```python
from build123d import *

# Parameters (mm, degrees)
ESQUISSE1_W                   = 32
ESQUISSE1_H                   = 100
BOSS_EXTRU_1_DEPTH            = 4
CHANFREIN1_SIZE               = 2.5
ESQUISSE2_W                   = 18
ESQUISSE2_H                   = 45
BOSS_EXTRU_2_DEPTH            = 32
ENL_V_MAT_EXTRU_1_DEPTH       = 151.159914758
ENL_V_MAT_EXTRU_1_DEPTH_BACK  = 151.159914758
ESQUISSE3_R                   = 3.25
ENL_V_MAT_EXTRU_2_DEPTH       = 143.91256068
ENL_V_MAT_EXTRU_2_DEPTH_BACK  = 143.91256068
ESQUISSE4_W                   = 55
ESQUISSE4_H                   = 32
ENL_V_MAT_EXTRU_3_DEPTH       = 117.292734081
ENL_V_MAT_EXTRU_3_DEPTH_BACK  = 117.292734081
ESQUISSE5_W                   = 45
ESQUISSE5_H                   = 23.5
CHANFREIN2_SIZE               = 6.5
ENL_V_MAT_EXTRU_4_DEPTH       = 5
ENL_V_START                   = 50
ENL_V_MAT_EXTRU_6_DEPTH       = 5
CONG_2_R                      = 3
ENL_V_MAT_EXTRU_7_DEPTH       = 151.159914758
ENL_V_MAT_EXTRU_7_DEPTH_BACK  = 151.159914758
CONG_3_R                      = 8
BOSS_EXTRU_3_DEPTH            = 4
BOSS_EXTRU_4_DEPTH            = 68
ESQUISSE10_W                  = 45
ESQUISSE10_H                  = 10
ENL_V_MAT_EXTRU_8_DEPTH       = 143.070405081
ENL_V_MAT_EXTRU_9_DEPTH       = 143.070405081
ENL_V_MAT_EXTRU_9_DEPTH_BACK  = 143.070405081
ESQUISSE11_R                  = 2.75
ENL_V_MAT_EXTRU_10_DEPTH      = 143.91256068
ENL_V_MAT_EXTRU_10_DEPTH_BACK = 143.91256068
ESQUISSE12_W                  = 24
ESQUISSE12_H                  = 5
CONG_4_R                      = 10
CONG_5_R                      = 3


# Some blends are built 0.0001 mm under size
with BuildPart() as part:
    # Esquisse1 → Boss.-Extru.1 (new body)
    with BuildSketch(Plane.XY):
        with Locations((16, 50)):
            Rectangle(ESQUISSE1_W, ESQUISSE1_H)
    extrude(amount=BOSS_EXTRU_1_DEPTH)

    # Chanfrein1
    chanfrein1_edges = [part.edges().sort_by_distance(p)[0] for p in [
        (16, 0, 0),
    ]]
    chamfer(chanfrein1_edges, length=CHANFREIN1_SIZE)

    # Esquisse2 → Boss.-Extru.2 (add)
    with BuildSketch(Plane(origin=(0, 0, 0), x_dir=(-1, 0, 0), z_dir=(0, 0, -1))):
        with Locations((-41, 107.5)):
            Rectangle(ESQUISSE2_W, ESQUISSE2_H)
        with Locations((9, 107.5)):
            Rectangle(ESQUISSE2_W, ESQUISSE2_H)
    extrude(amount=-BOSS_EXTRU_2_DEPTH)

    # Esquisse3 → Enlèv. mat.-Extru.1 (cut, two sides: drawn at the far end of the back side and taken through both)
    with BuildSketch(Plane.ZY.offset(18).offset(-ENL_V_MAT_EXTRU_1_DEPTH_BACK)):
        with Locations((21.5, 109.5)):
            Circle(ESQUISSE3_R)
    extrude(amount=ENL_V_MAT_EXTRU_1_DEPTH + ENL_V_MAT_EXTRU_1_DEPTH_BACK, mode=Mode.SUBTRACT)

    # Esquisse4 → Enlèv. mat.-Extru.2 (cut, two sides: drawn at the far end of the back side and taken through both)
    with BuildSketch(Plane.XY.offset(32).offset(-ENL_V_MAT_EXTRU_2_DEPTH_BACK)):
        with Locations((16, 116)):
            Rectangle(ESQUISSE4_W, ESQUISSE4_H)
    extrude(amount=ENL_V_MAT_EXTRU_2_DEPTH + ENL_V_MAT_EXTRU_2_DEPTH_BACK, mode=Mode.SUBTRACT)

    # Esquisse5 → Enlèv. mat.-Extru.3 (cut, two sides: drawn at the far end of the back side and taken through both)
    with BuildSketch(Plane(origin=(0, 100, 0), x_dir=(1, 0, 0), z_dir=(0, 1, 0)).offset(-ENL_V_MAT_EXTRU_3_DEPTH_BACK)):
        with Locations((16, -22.25)):
            Rectangle(ESQUISSE5_W, ESQUISSE5_H)
    extrude(amount=ENL_V_MAT_EXTRU_3_DEPTH + ENL_V_MAT_EXTRU_3_DEPTH_BACK, mode=Mode.SUBTRACT)

    # Chanfrein2
    chanfrein2_edges = [part.edges().sort_by_distance(p)[0] for p in [
        (0, 92.5, 10.5),
        (32, 92.5, 10.5),
    ]]
    chamfer(chanfrein2_edges, length=CHANFREIN2_SIZE - 0.0001)  # a hair under: the kernel refuses the full size

    # Esquisse6 → Enlèv. mat.-Extru.4 (cut)
    with BuildSketch(Plane(origin=(-6.5, 0, 0), x_dir=(0, 0, -1), z_dir=(1, 0, 0))):
        with BuildLine():
            Line((-28, 100), (-16, 100))
            ThreePointArc((-16, 100), (-22, 94), (-28, 100))
        make_face()
    extrude(amount=-ENL_V_MAT_EXTRU_4_DEPTH, mode=Mode.SUBTRACT)

    # Esquisse6<2> → Enlèv. mat.-Extru.6 (cut)
    with BuildSketch(Plane(origin=(-6.5, 0, 0), x_dir=(0, 0, -1), z_dir=(1, 0, 0)).offset(ENL_V_START)):
        with BuildLine():
            Line((-28, 100), (-16, 100))
            ThreePointArc((-16, 100), (-22, 94), (-28, 100))
        make_face()
    extrude(amount=-ENL_V_MAT_EXTRU_6_DEPTH, mode=Mode.SUBTRACT)

    # Congé2
    cong_2_edges = [part.edges().sort_by_distance(p)[0] for p in [
        (-9, 100, 16),
        (-9, 100, 28),
        (41, 100, 16),
        (41, 100, 28),
    ]]
    fillet(cong_2_edges, radius=CONG_2_R)

    # Esquisse7 → Enlèv. mat.-Extru.7 (cut, two sides: drawn at the far end of the back side and taken through both)
    with BuildSketch(Plane(origin=(50, 0, 0), x_dir=(0, 0, -1), z_dir=(1, 0, 0)).offset(-ENL_V_MAT_EXTRU_7_DEPTH_BACK)):
        Polygon((0, 100), (-18, 130), (0, 130), align=None)
    extrude(amount=ENL_V_MAT_EXTRU_7_DEPTH + ENL_V_MAT_EXTRU_7_DEPTH_BACK, mode=Mode.SUBTRACT)

    # Congé3
    cong_3_edges = [part.edges().sort_by_distance(p)[0] for p in [
        (46.75, 130, 18),
        (-14.75, 130, 18),
        (-14.75, 130, 32),
        (46.75, 130, 32),
    ]]
    fillet(cong_3_edges, radius=CONG_3_R)

    # Esquisse8 → Boss.-Extru.3 (add)
    with BuildSketch(Plane(origin=(0, 0, 0), x_dir=(-1, 0, 0), z_dir=(0, 0, -1))):
        Polygon((0, 55), (18, 85), (0, 85), align=None)
        Polygon((-32, 85), (-32, 55), (-50, 85), align=None)
    extrude(amount=-BOSS_EXTRU_3_DEPTH)

    # Esquisse9 → Boss.-Extru.4 (add)
    with BuildSketch(Plane.ZY.offset(18)):
        Polygon((32, 85), (4, 85), (4, 75), align=None)
    extrude(amount=-BOSS_EXTRU_4_DEPTH)

    # Esquisse10 → Enlèv. mat.-Extru.8 (cut, through all)
    with BuildSketch(Plane.XY.offset(4)):
        with Locations((16, 80)):
            Rectangle(ESQUISSE10_W, ESQUISSE10_H)
        Polygon((44, 75), (50, 85), (50, 75), align=None)
        Polygon((-12, 75), (-18, 85), (-18, 75), align=None)
    extrude(amount=ENL_V_MAT_EXTRU_8_DEPTH, mode=Mode.SUBTRACT)

    # Esquisse11 → Enlèv. mat.-Extru.9 (cut, two sides: drawn at the far end of the back side and taken through both)
    with BuildSketch(Plane.XY.offset(4).offset(-ENL_V_MAT_EXTRU_9_DEPTH_BACK)):
        with Locations((16, 45)):
            Circle(ESQUISSE11_R)
    extrude(amount=ENL_V_MAT_EXTRU_9_DEPTH + ENL_V_MAT_EXTRU_9_DEPTH_BACK, mode=Mode.SUBTRACT)

    # Esquisse12 → Enlèv. mat.-Extru.10 (cut, two sides: drawn at the far end of the back side and taken through both)
    with BuildSketch(Plane(origin=(0, 0, 0), x_dir=(-1, 0, 0), z_dir=(0, 0, -1)).offset(-ENL_V_MAT_EXTRU_10_DEPTH_BACK)):
        with Locations((-16, 97.5)):
            Rectangle(ESQUISSE12_W, ESQUISSE12_H)
    extrude(amount=ENL_V_MAT_EXTRU_10_DEPTH + ENL_V_MAT_EXTRU_10_DEPTH_BACK, mode=Mode.SUBTRACT)

    # Congé4
    # the kernel refuses this fillet: 10 mm, written as the material it adds along each edge
    with BuildSketch(Plane(origin=(4, 95, 0), x_dir=(0, 1, 0), z_dir=(0, 0, 1))) as cong_4_piece_1:
        with BuildLine():
            CenterArc((10, -8.660254038), CONG_4_R, 120, 60)
            Line((0, -8.660254038), (-0.2, -8.660254038))
            Line((-0.2, -8.660254038), (-0.2, 0))
            Line((-0.2, 0), (0, 0.2))
            ThreePointArc((0, 0.2), (2.5, 0.2), (4.9, 0.173205081))
            Line((4.9, 0.173205081), (5, 0))
        make_face()
    extrude(amount=4)
    with BuildSketch(Plane(origin=(28, 95, 4), x_dir=(-1, 0, 0), z_dir=(0, 0, -1))) as cong_4_piece_2:
        with BuildLine():
            CenterArc((8.660254038, 10), CONG_4_R, 210, 60)
            Line((0, 5), (-0.173205081, 4.9))
            ThreePointArc((-0.173205081, 4.9), (-0.2, 2.5), (-0.2, 0))
            Line((-0.2, 0), (0, -0.2))
            Line((0, -0.2), (8.660254038, -0.2))
            Line((8.660254038, -0.2), (8.660254038, 0))
        make_face()
    extrude(amount=4)

    # Congé5
    cong_5_edges = [part.edges().sort_by_distance(p)[0] for p in [
        (28, 100, 2),
        (4, 100, 2),
    ]]
    fillet(cong_5_edges, radius=CONG_5_R)


solid = part.part
```
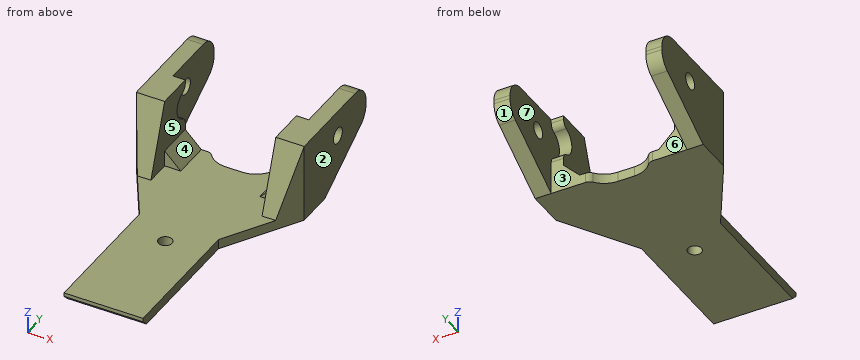
Work out the finished part from the listing and answer in its coordinate system (mm). Face numbers are marked on the shaded views. A direction names the side the tool comes from. Give positions to 0.01 mm unless a question says otherwise; leave off trailing zeros. Loops run counter-clockwise (first coordinate to the right, second up) from the corner with the lowest first, then second, coordinate; pieces in that order, holes last. Notation, with made-up numbers: (73, 37) -> (129, 37) arc R16 cw to (129, 58) -> close; hole circle Ø2 at (-34.5, 79). An arc over 180 degrees is marked (long way). One line per question, with ' | ' between items. Start each with the question number.
1) Section D-D, the plane z = 6.5 is taken. Determine the outline of the cut face in (x, y).
2) Section A-A, the plane x = 16 is taken. Determine the outline of the cut face in (y, z), then the cut area to 3 significant figures.
3) Determine the mould class of the marked faces 1, 2 and 3 for opening direction X: +X half, -X half, draft (parallel to the pull), parting line (faces both ways), or undercut.
4) Each of these flat-tipped pins is pushed along its axis until it touches: pin 1 (1.5 mm diameter, centred on x = -3.5, z = 10.5, fed in from -Y); pin 2 (7 mm diameter, centred on x = -4, z = 8.5, fed in from -Y); pin 3 (2 mm diameter, centred on x = 34, y = 76.5, fed in from +Z); pin 4 (1.2 mm diameter, centred on x = -8, z = 31.5, fed in from +Y). Where does it stop, or does it pass through?
5) Straight lines are drawn through the part: L1, parallel to X at y = 121, z = 23.5; L2, parallel to Z at x = 8.5, y = 53; L3, parallel to Y at x = -14, z = 21. For each, find the intervals that lie inside material, in ascending order.
6) For the marked faces 4, 5, 6 and 7, determine the directions among +Z, -Z, +X, -X, +Y, -Y from which every point of the face is accessible in a straight line to the end or side of a thin tool.
7) Section B-B, the plane y = 45 is taken. Determine the outline of the cut face in (x, z).
8) Section C-C, the plane y = 109.5 is taken. Determine the outline of the cut face in (x, z), then the cut area to 3 significant figures.
Resolved:
1) outline: (-18, 85) -> (-12.54, 75.89) -> (-6.5, 75.89) -> (-6.5, 85) -> (-2.5, 85) -> (-2.5, 100) -> (-11.5, 100) -> (-11.5, 110.83) -> (-18, 110.83) -> close; (34.5, 85) -> (38.5, 85) -> (38.5, 75.89) -> (44.54, 75.89) -> (50, 85) -> (50, 110.83) -> (43.5, 110.83) -> (43.5, 100) -> (34.5, 100) -> close
2) outline: (0, 2.5) -> (2.5, 0) -> (42.25, 0) -> (42.25, 4) -> (0, 4) -> close; (47.75, 0) -> (95, 0) -> (95, 4) -> (47.75, 4) -> close | area: 355 mm2
3) face 1: draft | face 2: +X half | face 3: undercut
4) pin 1: through | pin 2: y = 75.73 | pin 3: z = 4 | pin 4: y = 100
5) L1: -18 to -11.5, 43.5 to 50 | L2: 0 to 4 | L3: 81.07 to 106.29, 112.71 to 129.85
6) face 4: +Z, +Y, -Y | face 5: +Z, -Y | face 6: +Z, -Z, +Y | face 7: +Y
7) outline: (0, 0) -> (13.25, 0) -> (13.25, 4) -> (0, 4) -> close; (18.75, 0) -> (32, 0) -> (32, 4) -> (18.75, 4) -> close
8) outline: (-18, 5.7) -> (-11.5, 5.7) -> (-11.5, 18.25) -> (-18, 18.25) -> close; (-18, 24.75) -> (-11.5, 24.75) -> (-11.5, 32) -> (-18, 32) -> close; (43.5, 5.7) -> (50, 5.7) -> (50, 18.25) -> (43.5, 18.25) -> close; (43.5, 24.75) -> (50, 24.75) -> (50, 32) -> (43.5, 32) -> close | area: 257 mm2
